Check sheet for the modelled part. Datum: model origin and axes. Units: mm. A direction names the side the tool comes from. Round coordinates to 2 decimals unless told otherwise and drop trailing zeros. Write each loop counter-clockwise with the first axis right and the second up, starting at its lowest first coordinate (ties: lowest second). Pieces come first, ordered by that corner, then holes. Notation, with made-up numbers: (4.25, 18.25) -> (49.25, 18.25) arc R36 cw to (49.25, 54.25) -> close; hole circle Ø5 at (25, 6). An arc over 180 degrees is marked (long way). Answer as a JSON object with one key per item and string values. Group by question number.
```python
from build123d import *

# Parameters (mm, degrees)
F0_W     = 24
F0_H     = 10
F0_H_2   = 2
F0_W_2   = 2
F0_W_3   = 22
F1_DEPTH = 2
F2_DEPTH = 4


with BuildPart() as f1:
    # F0 (on Top) → F1 (new body)
    with BuildSketch(Plane.XY):
        with Locations((-13, 0)):
            Rectangle(F0_W, F0_H)
        with Locations((-13, -6)):
            Rectangle(F0_W, F0_H_2)
        Rectangle(F0_W_2, F0_H)
        with Locations((12, -6)):
            Rectangle(F0_W_3, F0_H_2)
        with Locations((24, -6)):
            Rectangle(F0_W_2, F0_H_2)
        with Locations((24, 0)):
            Rectangle(F0_W_2, F0_H)
        with Locations((12, 0)):
            Rectangle(F0_W_3, F0_H)
        with Locations((12, 6)):
            Rectangle(F0_W_3, F0_H_2)
        with Locations((-13, 6)):
            Rectangle(F0_W, F0_H_2)
        with Locations((24, 6)):
            Rectangle(F0_W_2, F0_H_2)
    extrude(amount=F1_DEPTH)

    # F0 (on Top) → F2 (join)
    with BuildSketch(Plane.XY):
        with Locations((12, -6)):
            Rectangle(F0_W_3, F0_H_2)
        with Locations((24, -6)):
            Rectangle(F0_W_2, F0_H_2)
        with Locations((24, 0)):
            Rectangle(F0_W_2, F0_H)
        with Locations((24, 6)):
            Rectangle(F0_W_2, F0_H_2)
        with Locations((12, 6)):
            Rectangle(F0_W_3, F0_H_2)
        with Locations((-13, 6)):
            Rectangle(F0_W, F0_H_2)
        with Locations((-13, -6)):
            Rectangle(F0_W, F0_H_2)
    extrude(amount=F2_DEPTH)


solid = f1.part
```
(1) Section check A-A on y = -6. Record the cut outline in (x, z), then the cut area to 3 significant figures.
(2) Section check D-D on y = -1.5. Record the cut outline in (x, z), then the cut area to 3 significant figures.
(3) Go/stop test with flat-tipped pins: pin 1 Ø1 at (x, z) = (0, 1.5) entering from -Y; pin 2 Ø1 at (y, z) = (-2, 3) entering from -X; pin 3 Ø3 at (x, y) = (7.5, -2.5) entering from +Z. Record where each tip stops, or that it passes through.
(4) Access from +Z, -Z, +X, -X, +Y, -Y to the whole of each face (thin tool, end or side, straight path). Record for faces 1 (the flat face through (1, 6, 2)), 2 (the flat face through (-13, 7, 2)), 3 (the flat face through (12, -5, 3)), 4 (the flat face through (0, -5, 1)).
(5) Scan lines: line 1 along X through (y, z) = (-6.5, 2.9); line 2 along Y through (x, z) = (-6.5, 2.3); line 3 along X through (y, z) = (-4.25, 2.35). Record each from-to range of solid material in increasing order.
(6) Section check B-B on z = 2.75. Record the cut outline in (x, y), then the cut area to 3 significant figures.
(7) Release check for a two-part mould opening along Y. For faces 5 (the flat face through (12, 5, 3)), 6 (the flat face through (13, 7, 2)), 7 (the flat face through (-1, -6, 2)), 8 (the flat face through (-13, 5, 3)) record: pulls with the +Y half, pulls with the -Y half, needs draft (parallel to the pull), parting line crosses it, or undercut.
(8) Section check C-C on x = -18. Record the cut outline in (y, z), then the cut area to 3 significant figures.
Data:
{
 "1": {"outline": "(-25, 0) -> (-1, 0) -> (-1, 4) -> (-25, 4) -> close; (1, 0) -> (25, 0) -> (25, 4) -> (1, 4) -> close", "area": "192 mm²"},
 "2": {"outline": "(-25, 0) -> (25, 0) -> (25, 4) -> (23, 4) -> (23, 2) -> (-25, 2) -> close", "area": "104 mm²"},
 "3": {"pin 1": "stops at y = -5", "pin 2": "stops at x = 23", "pin 3": "stops at z = 2"},
 "4": {"face 1": "+Z, -Z, +Y", "face 2": "+Z, -Z, +X, -X, +Y", "face 3": "+Z, -X", "face 4": "+Z, -Z, -Y"},
 "5": {"line 1": "x = -25 to -1, 1 to 25", "line 2": "y = -7 to -5, 5 to 7", "line 3": "x = 23 to 25"},
 "6": {"outline": "(-25, -7) -> (-1, -7) -> (-1, -5) -> (-25, -5) -> close; (-25, 5) -> (-1, 5) -> (-1, 7) -> (-25, 7) -> close; (1, -7) -> (25, -7) -> (25, 7) -> (1, 7) -> (1, 5) -> (23, 5) -> (23, -5) -> (1, -5) -> close", "area": "212 mm²"},
 "7": {"face 5": "undercut", "face 6": "pulls with the +Y half", "face 7": "needs draft", "face 8": "undercut"},
 "8": {"outline": "(-7, 0) -> (7, 0) -> (7, 4) -> (5, 4) -> (5, 2) -> (-5, 2) -> (-5, 4) -> (-7, 4) -> close", "area": "36.0 mm²"}
}
